Geometry check sheet. Reference: the model listing, model coordinates, mm. Face numbers are marked on the shaded views. Coordinates: 2 decimals unless noted, no trailing zeros. Order: outer loops, then holes, each group sorted by start corner. A loop starts at its lowest first (then second) coordinate and runs counter-clockwise, first axis right, second up. Notation, with made-up numbers: (37, 80.5) - (49, 80.5) arc R15 ccw to (49, 97.5) - close; hole circle Ø3 at (18.25, -36). An arc over 180 degrees is marked (long way). Return JSON: item names as keys, results as strings. Group by question number.
Item 1: Draft check along X on the marked faces 1, 2 and 3. Enter one of: pulls with the +X half, pulls with the -X half, needs draft (parallel to the pull), parting line crosses it, or undercut.
Item 2: Gauge pin test, flat end, axial feed: pin 1 (5 mm diameter, centred on x = -11.5, y = -4, fed in from +Z). Record the tip position at first contact, or that the pin passes through.
Item 3: Section check B-B on z = 0.7. Enter the section's corners in (x, y), then the cut area to 3 significant figures.
Item 4: Section check D-D on x = 0. Enter the section's corners in (y, z), then the cut area to 3 significant figures.
Item 5: Section check A-A on y = -13.5. Enter the section's corners in (x, z), then the cut area to 3 significant figures.
Item 6: Scan lines: probe 1 along X at (y, z) = (-11.5, -0.7); probe 2 along X at (y, z) = (-11.75, 0); probe 3 along Y at (x, z) = (-6, -1.2). Record each from-to range of solid material in increasing order.
Item 7: Section check C-C on y = -10.75. Enter the section's corners in (x, z), then the cut area to 3 significant figures.
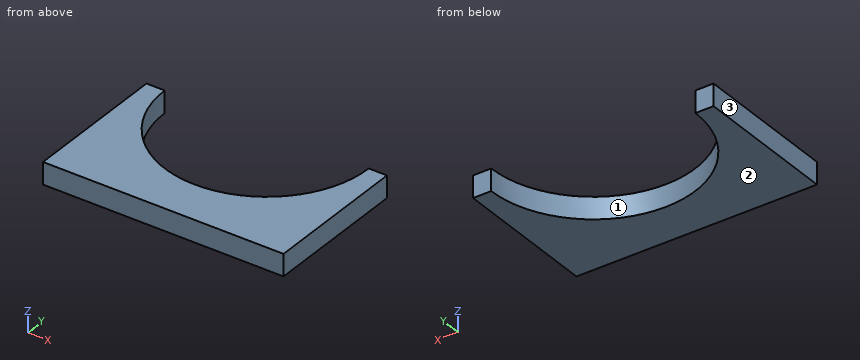
from build123d import *

# Parameters (mm, degrees)
BOSS_EXTRUDE1_DEPTH = 1.5


with BuildPart() as part:
    # Sketch1 → Boss-Extrude1 (new, symmetric)
    with BuildSketch(Plane.XY):
        with BuildLine():
            Line((-16.5, 0), (-14, 0))
            ThreePointArc((-14, 0), (0, -14), (14, 0))
            Line((14, 0), (16.5, 0))
            Line((16.5, 0), (16.5, -20))
            Line((16.5, -20), (-16.5, -20))
            Line((-16.5, -20), (-16.5, 0))
        make_face()
    extrude(amount=BOSS_EXTRUDE1_DEPTH, both=True)


solid = part.part
Computed:
{
 "1": {"face 1": "undercut", "face 2": "needs draft", "face 3": "pulls with the -X half"},
 "2": {"pin 1": "stops at z = 1.5"},
 "3": {"outline": "(-16.5, -20) - (16.5, -20) - (16.5, 0) - (14, 0) arc R14 cw to (-14, 0) - (-16.5, 0) - close", "area": "352 mm²"},
 "4": {"outline": "(-20, -1.5) - (-14, -1.5) - (-14, 1.5) - (-20, 1.5) - close", "area": "18.0 mm²"},
 "5": {"outline": "(-16.5, -1.5) - (-3.71, -1.5) - (-3.71, 1.5) - (-16.5, 1.5) - close; (3.71, -1.5) - (16.5, -1.5) - (16.5, 1.5) - (3.71, 1.5) - close", "area": "76.8 mm²"},
 "6": {"probe 1": "x = -16.5 to -7.98, 7.98 to 16.5", "probe 2": "x = -16.5 to -7.61, 7.61 to 16.5", "probe 3": "y = -20 to -12.65"},
 "7": {"outline": "(-16.5, -1.5) - (-8.97, -1.5) - (-8.97, 1.5) - (-16.5, 1.5) - close; (8.97, -1.5) - (16.5, -1.5) - (16.5, 1.5) - (8.97, 1.5) - close", "area": "45.2 mm²"}
}
